Verification items for the finished model (mm, model axes). A direction names the side the tool comes from. Coordinates: 2 decimals unless noted, no trailing zeros. Order: outer loops, then holes, each group sorted by start corner. A loop starts at its lowest first (then second) coordinate and runs counter-clockwise, first axis right, second up. Notation, with made-up numbers: M 54.5,-28.5 L 78.5,-28.5 A10 ccw 78.5,-12.5 Z; hole C 56,-8 d5. An arc over 180 degrees is marked long. Use one line per item in the form item = value. Start each with the question number.
```python
from build123d import *

# Parameters (mm, degrees)
F0_W     = 45
F0_H     = 45
F1_DEPTH = 275
F2_W     = 45
F2_H     = 13.5
F3_DEPTH = 45.001
F5_DEPTH = 45.001


# Not quite as in the source:
# - a pattern or mirror of a feature is missing from the dataset's text; its kind, count and spacing are read off the source's solid


with BuildPart() as f1:
    # F0 (on Right) → F1 (new body, symmetric)
    with BuildSketch(Plane.YZ):
        Rectangle(F0_W, F0_H)
    extrude(amount=F1_DEPTH, both=True)

    # F2 (on face) → F3 (cut, through all)
    with BuildSketch(Plane.XY.offset(22.5)):
        with Locations((0, 15.75)):
            Rectangle(F2_W, F2_H)
        with Locations((0, -15.75)):
            Rectangle(F2_W, F2_H)
    extrude(amount=-F3_DEPTH, mode=Mode.SUBTRACT)

    # F4 (on face) → F5 (cut, through all)
    with BuildSketch(Plane.XZ.offset(22.5)):
        Polygon((275, 22.5), (213.1817580623, 22.5), (275, 0), align=None)
    f5 = extrude(amount=-F5_DEPTH, mode=Mode.SUBTRACT)

    # F5_copies: F5 across plane
    add(f5.mirror(Plane(origin=(0, 0, 0), x_dir=(0, 0, -1), z_dir=(-1, 0, 0))), mode=Mode.SUBTRACT)


solid = f1.part
```
1. Material ranges on line 1 along X through (y, z) = (-21, -7); line 2 along Z through (x, y) = (236, -15.5); line 3 along Z through (x, y) = (251, -17), recorded low to high.
2. Cross-section at B-B on y = -16. Enter the section's corners in (x, z).
3. Tool access check on faces 1 (the flat face through (22.5, -16, 0)), 2 (the flat face through (4, 0, -22.5)), 3 (the flat face through (22.5, 16, 0)). Record the directions out of +Z, -Z, +X, -X, +Y, -Y that give a thin tool (end or side, any length) a straight path to the whole face; none if there is none.
4. Cross-section at D-D on x = -218. Enter the section's corners in (y, z).
5. Cross-section at C-C on x = 1.5. Enter the section's corners in (y, z).
6. Cross-section at A-A on z = -15. Enter the section's corners in (x, y), and give its area (3 significant figures).
7. Depth check by flat-ended pin: P1, Ø22.5, axis at x = -10.5, z = 5, coming from the -Y side. Enter the tip coordinate at first touch or a pass-through.
8. Release check for a two-part mould opening along X. For faces 4 (the flat face through (275, 0, -11)), 5 (the flat face through (-147, 22.5, 0)), 6 (the flat face through (-22.5, -16, 0)) record: pulls with the +X half, pulls with the -X half, needs draft (parallel to the pull), parting line crosses it, or undercut.
Final values:
q1.line_1 = -275 to -22.5, 22.5 to 275
q1.line_2 = -22.5 to 14.19
q1.line_3 = -22.5 to 8.74
q2.outline = M -275,-22.5 L -22.5,-22.5 L -22.5,22.5 L -213.18,22.5 L -275,0 Z; M 22.5,-22.5 L 275,-22.5 L 275,0 L 213.18,22.5 L 22.5,22.5 Z
q3.face_1 = +Z, -Z, -Y
q3.face_2 = -Z, +X, -X, +Y, -Y
q3.face_3 = +Z, -Z, +Y
q4.outline = M -22.5,-22.5 L 22.5,-22.5 L 22.5,20.75 L -22.5,20.75 Z
q5.outline = M -9,-22.5 L 9,-22.5 L 9,22.5 L -9,22.5 Z
q6.outline = M -275,-22.5 L -22.5,-22.5 L -22.5,-9 L 22.5,-9 L 22.5,-22.5 L 275,-22.5 L 275,22.5 L 22.5,22.5 L 22.5,9 L -22.5,9 L -22.5,22.5 L -275,22.5 Z
q6.area = 23,500 mm2
q7.P1 = -9
q8.face_4 = pulls with the +X half
q8.face_5 = needs draft
q8.face_6 = undercut
